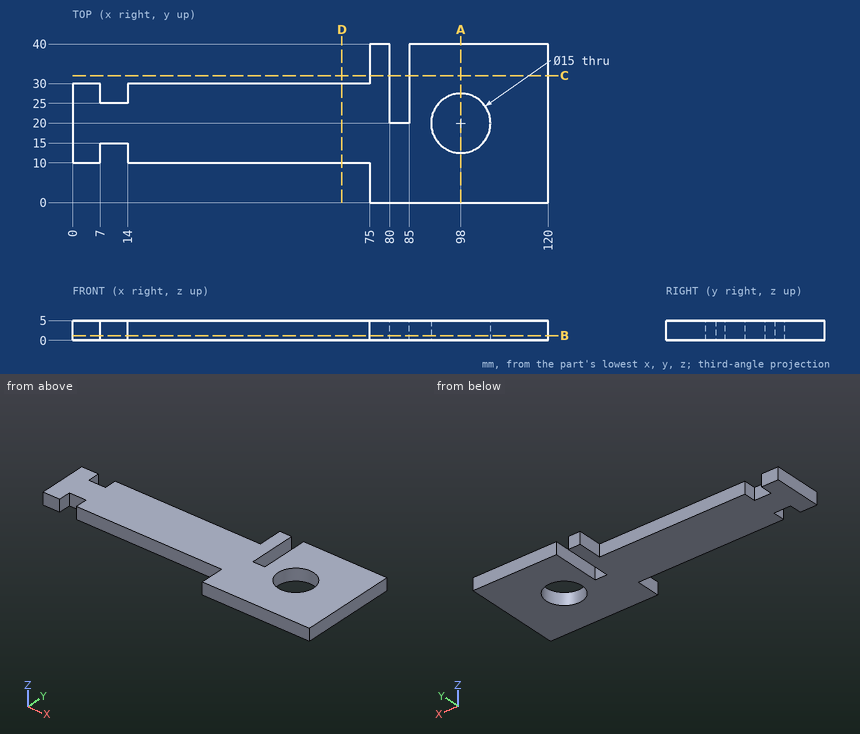
Input: dimensioned drawing with shaded views. Units: mm. Origin: part minimum x, y, z. Give positions to 0.01 mm unless a question says otherwise; leave off trailing zeros. Loops run counter-clockwise (first coordinate to the right, second up) from the corner with the lowest first, then second, coordinate; pieces in that order, holes last. Notation, with made-up numbers: (62.25, -13) -> (99.25, -13) arc R7 ccw to (99.25, -5) -> close; hole circle Ø6 at (36, 36). An arc over 180 degrees is marked (long way). Use a Markdown table: item, result.
Q1. First-contact query: P1, Ø1.5, axis at x = 30, z = 3, coming from the -Y side; P2, Ø1.5, axis at y = 5.5, z = 2, coming from the -X side; P3, Ø1.5, axis at x = 10, z = 2.5, coming from the -Y side; P4, Ø12, axis at x = 98, y = 20, coming from the -Z side. Flat tips, straight axial feed; report the tip coordinate or a pass-through.
Entries:
| item | result |
|---|---|
| P1 | stops at y = 10 |
| P2 | stops at x = 75 |
| P3 | stops at y = 15 |
| P4 | passes through |
Q2. Section query B-B, the plane z = 1.2. Return the cut outline in (x, y).
Entries:
| item | result |
|---|---|
| outline | (0, 10) -> (7, 10) -> (7, 15) -> (14, 15) -> (14, 10) -> (75, 10) -> (75, 0) -> (120, 0) -> (120, 40) -> (85, 40) -> (85, 20) -> (80, 20) -> (80, 40) -> (75, 40) -> (75, 30) -> (14, 30) -> (14, 25) -> (7, 25) -> (7, 30) -> (0, 30) -> close; hole circle Ø15 at (98, 20) |
Q3. Section query D-D, the plane x = 68. Return the cut outline in (y, z).
Entries:
| item | result |
|---|---|
| outline | (10, 0) -> (30, 0) -> (30, 5) -> (10, 5) -> close |
Q4. Section query C-C, the plane y = 32. Return the cut outline in (x, z).
Entries:
| item | result |
|---|---|
| outline | (75, 0) -> (80, 0) -> (80, 5) -> (75, 5) -> close; (85, 0) -> (120, 0) -> (120, 5) -> (85, 5) -> close |
Q5. Ray query, probe 1 along X at (y, z) = (28, 3.9); probe 2 along X at (y, z) = (20.5, 2.1); probe 3 along Y at (x, z) = (98, 2.6). Return the intervals inside material, ascending. Write a range as from..to.
Entries:
| item | result |
|---|---|
| probe 1 | x = 0..7, 14..80, 85..120 |
| probe 2 | x = 0..80, 85..90.52, 105.48..120 |
| probe 3 | y = 0..12.5, 27.5..40 |
Q6. Section query A-A, the plane x = 98. Return the cut outline in (y, z).
Entries:
| item | result |
|---|---|
| outline | (0, 0) -> (12.5, 0) -> (12.5, 5) -> (0, 5) -> close; (27.5, 0) -> (40, 0) -> (40, 5) -> (27.5, 5) -> close |
